Autodesk Fusion 360 part; units mm, degrees
sketch "Sketch1" plane through (0, 0, 0) normal (0, 0, 1) x (1, 0, 0)
  line L0 (-13.5, 19) -> (13.5, 19)
  line L1 (13.5, 19) -> (13.5, -19)
  line L2 (13.5, -19) -> (-13.5, -19)
  line L3 (-13.5, -19) -> (-13.5, 19)
  line L4 (-13.5, 19) -> (13.5, -19) construction
  line L5 (14.5, -20) -> (-14.5, -20)
  line L6 (-14.5, -20) -> (-14.5, 20)
  line L7 (-14.5, 20) -> (14.5, 20)
  line L8 (14.5, 20) -> (14.5, -20)
  line L9 (-45, 45) -> (45, 45)
  line L10 (45, 45) -> (45, -45)
  line L11 (45, -45) -> (-45, -45)
  line L12 (-45, -45) -> (-45, 45)
  line L13 (-45, 45) -> (45, -45) construction
  line L14 (-14.5, -20) -> (-45, -45)
  line L15 (-14.5, 20) -> (-45, 45)
  line L16 (14.5, 20) -> (45, 45)
  line L17 (14.5, -20) -> (45, -45)
  line L18 (-43.5, 43.5) -> (43.5, 43.5)
  line L19 (43.5, 43.5) -> (43.5, -43.5)
  line L20 (43.5, -43.5) -> (-43.5, -43.5)
  line L21 (-43.5, -43.5) -> (-43.5, 43.5)
  line L22 (-12.9225, 20) -> (-41.5925, 43.5)
  line L23 (-14.5, 18.707) -> (-43.5, 42.4775)
  line L24 (14.5, 18.707) -> (43.5, 42.4775)
  line L25 (12.9225, 20) -> (41.5925, 43.5)
  line L26 (12.9225, -20) -> (41.5925, -43.5)
  line L27 (14.5, -18.707) -> (43.5, -42.4775)
  line L28 (-14.5, -18.707) -> (-43.5, -42.4775)
  line L29 (-12.9225, -20) -> (-41.5925, -43.5)
  dimension "d5" = 27
  dimension "d6" = 38
  dimension "d15" = 90
  dimension "d16" = 90
  dimension "d44" = 1.5
ref_plane "WorkPlane1" through (0, 0, 85) normal (0, 0, 1) x (1, 0, 0)
sketch "Sketch2" plane through (0, 0, 85) normal (0, 0, 1) x (1, 0, 0)
  circle A0 centre (0, 0) radius 28.425
  circle A1 centre (0, 0) radius 30.325
  circle A2 centre (0, 0) radius 27.925
  circle A3 centre (0, 0) radius 30.825
  dimension "d10" = 56.85
  dimension "d11" = 60.65
  dimension "d13" = -0.5
  dimension "d14" = 0.5
loft "Loft3" add profiles "Sketch1", "Sketch2" section 1 contours L5 L6 L7 L8 section 2 contours A0 | A1 | A3 makes body 1
loft "Loft4" cut profiles "Sketch2", "Sketch1" section 1 contours A2 section 2 contours L0 L1 L2 L3 bodies 1
extrude "Extrude3" add sketch "Sketch1" along normal blind 1.5 separate body contours L5 L17 L20 L26 | L8 L17 L19 L20 L27 | L5 L20 L26 L29 | L8 L19 L24 L27 | L10 L16 L17 L18 L19 L20 | L11 L14 L17 L20 | L5 L14 L20 L29 | L8 L16 L18 L19 L24 | L6 L14 L20 L21 L28 | L7 L16 L18 L25 | L9 L15 L16 L18 | L12 L14 L15 L18 L20 L21 | L6 L21 L23 L28 | L7 L18 L22 L25 | L6 L15 L18 L21 L23 | L7 L15 L18 L22 makes body 2
extrude "Extrude4" add sketch "Sketch2" along normal blind 7 bodies 1
extrude "Extrude7" add sketch "Sketch1" along normal blind 3 contours L5 L17 L20 L26 | L8 L17 L19 L20 L27 | L10 L16 L17 L18 L19 L20 | L11 L14 L17 L20 | L5 L14 L20 L29 | L8 L16 L18 L19 L24 | L6 L14 L20 L21 L28 | L7 L16 L18 L25 | L9 L15 L16 L18 | L12 L14 L15 L18 L20 L21 | L6 L15 L18 L21 L23 | L7 L15 L18 L22 bodies 1 2
fillet "Fillet1" radius 3 4 edges at (45, -45, 1.5) (-45, -45, 1.5) (-45, 45, 1.5) (45, 45, 1.5) on bodies 1
equation "aparture_x = 27 mm"
equation "aparture_y = 38 mm"
equation "tube_height = 85 mm"
equation "hood_lip_wall_thickness = 1 mm"
equation "d5 = aparture_x"
equation "d6 = aparture_y"
equation "d7 = tube_height"
equation "hood_inner_dia = 57 mm"
equation "hood_outer_dia = 60.5 mm"
equation "d10 = hood_inner_dia - hood_tolerance / 2"
equation "d11 = hood_outer_dia + hood_tolerance / 2"
equation "d13 = -hood_lip_wall_thickness / 2"
equation "d14 = hood_lip_wall_thickness / 2"
equation "d15 = raft_y"
equation "d16 = raft_x"
equation "raft_height = 1.5 mm"
equation "d22 = raft_height"
equation "hood_lip_height = 7 mm"
equation "d25 = hood_lip_height"
equation "raft_x = 90 mm"
equation "raft_y = 90 mm"
equation "rib_width = 1.5 mm"
equation "d44 = rib_width"
equation "rib_height = 1.5 mm"
equation "d54 = raft_height + rib_height"
equation "round_corner_radius = 3 mm"
equation "d58 = round_corner_radius"
equation "hood_tolerance = 0.3 mm"
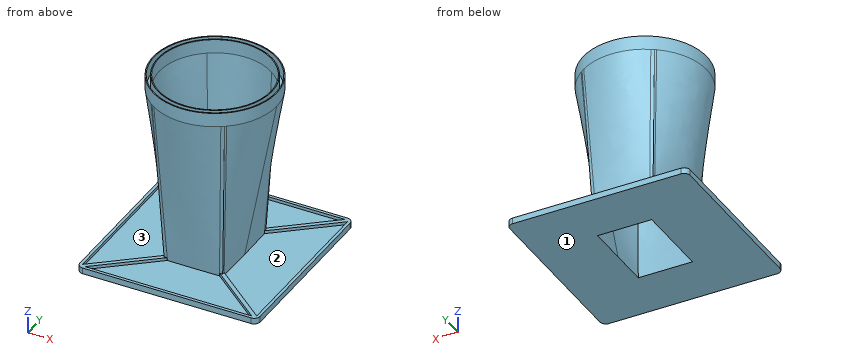
CAD build for the part. Positions are in the model's coordinates, mm. Face numbers are marked on the shaded views. Coordinates: 2 decimals unless noted, no trailing zeros. Loops run counter-clockwise (first coordinate to the right, second up) from the corner with the lowest first, then second, coordinate; pieces in that order, holes last. Notation, with made-up numbers: (-5, -20) - (1, -20) arc R31 ccw to (1, 11) - close; hole circle Ø7 at (44, -11). An arc over 180 degrees is marked (long way). Write item = value, one per line. Start each with the question number.
Q1. Cut at A-A, the plane x = 37.5. List the corners of the cut face in (y, z).
Q2. Drill centre lines: L1, parallel to Y at x = 0, z = 87.75 (3 decimals); L2, parallel to Z at x = -15, y = 35; L3, parallel to Y at x = -11, z = 74. Where is each one in solid material? Low to high.
Q3. Flat gauge pins, fed straight in: pin 1 Ø6 at (x, y) = (9, -13) entering from +Z (1 decimal); pin 2 Ø3 at (y, z) = (-3.5, 29) entering from -X; pin 3 Ø4 at (x, z) = (-5.5, 77.5) entering from -Y; pin 4 Ø12 at (y, z) = (-11, 82.5) entering from +X. Where does each tip first touch, or does it go through?
Q4. Pull direction Y, two halves, no side cores. Call the marked faces 1, 2 and 3: pulls with the +Y half, pulls with the -Y half, needs draft (parallel to the pull), parting line crosses it, or undercut.
Computed:
q1.outline = (-45, 0) - (45, 0) - (45, 3) - (43.5, 3) - (43.5, 1.5) - (40.15, 1.5) - (40.15, 3) - (37.56, 3) - (37.56, 1.5) - (-37.56, 1.5) - (-37.56, 3) - (-40.15, 3) - (-40.15, 1.5) - (-43.5, 1.5) - (-43.5, 3) - (-45, 3) - close
q2.L1 = -30.825 to -30.325, -28.425 to -27.925, 27.925 to 28.425, 30.325 to 30.825
q2.L2 = 0 to 1.5
q2.L3 = -27.53 to -24.7, 24.7 to 27.53
q3.pin_1 = through
q3.pin_2 = -20.26
q3.pin_3 = -29.79
q3.pin_4 = 30.32
q4.face_1 = needs draft
q4.face_2 = undercut
q4.face_3 = undercut
